For this review, take the finished solid that the model builds, in its own axes (mm). A direction names the side the tool comes from. Coordinates: 2 decimals unless noted, no trailing zeros. Loops run counter-clockwise (first coordinate to the right, second up) from the corner with the lowest first, then second, coordinate; pieces in that order, holes last. Notation, with made-up numbers: (38.5, 1.25) - (88.5, 1.25) arc R24 ccw to (88.5, 20.25) - close; hole circle Ø6 at (6.25, 71.25). An arc over 180 degrees is marked (long way). Use one line per item in the form item = value. Start each with the question number.
1. Draft analysis for pull direction Y (two halves, no side actions). For faces 1 (the face through (28, -33, 0)), 2 (the face through (4, -70, 0)), 3 (the face through (1.267, -65.07, 1.341)), 4 (the face through (11, 6, 0)), state which applies: +Y half, -Y half, draft (parallel to the pull), parting line (faces both ways), or undercut.
2. To check wall thickness, follow probe 1 along X at (y, z) = (-17.5, 0.25); probe 2 along Y at (x, z) = (16, 6); probe 3 along Y at (x, z) = (5, -5.75). State the ranges of each line that lie inside material, in increasing order.
3. Add section A-A on x = 4.5. Give the boundary of the cut face in (y, z), and give its area (3 significant figures).
4. For pin 1 Ø1.5 at (x, z) = (5, 2.5) entering from +Y; pin 2 Ø6 at (y, z) = (-23.5, 4) entering from -X; pin 3 Ø4 at (x, z) = (-3.5, 0.5) entering from -Y, all flat-tipped, find the tip position at first contact; note any pin that passes through.
5. Machinability: for faces 5 (the face through (18, -40, 0)), 6 (the face through (0, -72, 0)), 7 (the face through (23, -24, 0)), which of the approach directions +Z, -Z, +X, -X, +Y, -Y give a long, thin tool a straight path to every point of the face, cutting with its end or side? Answer none if there is none.
6. Add section B-B on z = 0. Count the separate pieces of the cut face and the enclosed holes in it, and give its area (3 significant figures).
7. Add section D-D on y = -64.5. Give the boundary of the cut face in (x, z).
8. Add section C-C on y = -77.5. Give the boundary of the cut face in (x, z).
```python
from build123d import *

# Parameters (mm, degrees)
BOSS_EXTRUDE1_DEPTH          = 7.5
CUT_EXTRUDE1_REACH           = 158.924
SKETCH2_W                    = 18
SKETCH2_H                    = 40
M5_CLEARANCE_HOLE1_D         = 5.8
CUT_EXTRUDE2_REACH           = 158.924
F_7_0_7_DIAMETER_HOLE1_D     = 7
F_7_0_7_DIAMETER_HOLE1_DEPTH = 20
MOVE_FACE1_BY                = 0.6
CUT_EXTRUDE3_REACH           = 141.732
SKETCH14_W                   = 15
SKETCH14_H                   = 15
BOSS_EXTRUDE2_DEPTH          = 10
M5_CLEARANCE_HOLE2_D         = 5.8
SKETCH18_W                   = 33
SKETCH18_H                   = 15
SKETCH18_R                   = 5
BOSS_EXTRUDE3_DEPTH          = 6
SKETCH19_R                   = 5
SKETCH19_R_2                 = 2.9
BOSS_EXTRUDE4_DEPTH          = 1
F_7_0_7_DIAMETER_HOLE2_D     = 7
F_7_0_7_DIAMETER_HOLE2_DEPTH = 30


with BuildPart() as part:
    # Sketch1 → Boss-Extrude1 (new, symmetric)
    with BuildSketch(Plane.XY):
        Polygon((0, 0), (120, 0), (0, -100), align=None)
    extrude(amount=BOSS_EXTRUDE1_DEPTH, both=True)

    # Sketch2 → Cut-Extrude1 (cut, up to next)
    with BuildSketch(Plane.XY.offset(7.5), mode=Mode.PRIVATE) as cut_extrude1_sk1:
        with Locations((9, -40)):
            Rectangle(SKETCH2_W, SKETCH2_H)
    cut_extrude1_tool1 = extrude(cut_extrude1_sk1.sketch, amount=-CUT_EXTRUDE1_REACH, mode=Mode.PRIVATE) & part.part
    add(cut_extrude1_tool1.solids().sort_by_distance((9, -40, 7.5))[0], mode=Mode.SUBTRACT)

    # M5 Clearance Hole1 (through all)
    with Locations(Plane(origin=(0, 0, 0), x_dir=(1, 0, 0), z_dir=(0, 1, 0))):
        with Locations((4.5, 0)):
            Hole(M5_CLEARANCE_HOLE1_D / 2)

    # Sketch8 → Cut-Extrude2 (cut, up to next)
    with BuildSketch(Plane.XY.offset(7.5), mode=Mode.PRIVATE) as cut_extrude2_sk1:
        Polygon((0, -70), (36, -70), (0, -100), align=None)
    cut_extrude2_tool1 = extrude(cut_extrude2_sk1.sketch, amount=-CUT_EXTRUDE2_REACH, mode=Mode.PRIVATE) & part.part
    add(cut_extrude2_tool1.solids().sort_by_distance((12, -80, 7.5))[0], mode=Mode.SUBTRACT)

    # Ø7.0 (7) Diameter Hole1
    with Locations(Plane(origin=(0, 0, 0), x_dir=(1, 0, 0), z_dir=(0, 1, 0))):
        with Locations((60, 0)):
            Hole(F_7_0_7_DIAMETER_HOLE1_D / 2, depth=F_7_0_7_DIAMETER_HOLE1_DEPTH)

    # Move Face1: a curved face moved inward by 0.6
    add(Solid.thicken(part.faces().sort_by_distance((7.4, -65, 0))[0], -MOVE_FACE1_BY), mode=Mode.SUBTRACT)

    # Sketch13 → Cut-Extrude3 (cut, up to next)
    with BuildSketch(Plane.XY.offset(7.5), mode=Mode.PRIVATE) as cut_extrude3_sk1:
        Polygon((28, 0), (28, -70), (36, -70), (120, 0), align=None)
    cut_extrude3_tool1 = extrude(cut_extrude3_sk1.sketch, amount=-CUT_EXTRUDE3_REACH, mode=Mode.PRIVATE) & part.part
    add(cut_extrude3_tool1.solids().sort_by_distance((58.88, -25.2, 7.5))[0], mode=Mode.SUBTRACT)

    # Sketch14 → Boss-Extrude2 (add)
    with BuildSketch(Plane.ZY):
        with Locations((0, -77.5)):
            Rectangle(SKETCH14_W, SKETCH14_H)
    extrude(amount=-BOSS_EXTRUDE2_DEPTH)

    # M5 Clearance Hole2 (through all)
    with Locations(Plane(origin=(10, 0, 0), x_dir=(0, 0, -1), z_dir=(1, 0, 0))):
        with Locations((0, -77.5)):
            Hole(M5_CLEARANCE_HOLE2_D / 2)



with BuildPart() as body_2:
    # Sketch18 → Boss-Extrude3 (new body)
    with BuildSketch(Plane(origin=(0, 0, 0), x_dir=(1, 0, 0), z_dir=(0, 1, 0))):
        with Locations((11.5, 0)):
            Rectangle(SKETCH18_W, SKETCH18_H)
        with Locations(Location((4.5, 0, 0), (0, 0, 270))):
            Circle(SKETCH18_R, mode=Mode.SUBTRACT)
    extrude(amount=BOSS_EXTRUDE3_DEPTH)


with BuildPart() as part_1:
    add(part.part)

    add(body_2.part)  # Boss-Extrude4 merges body 2
    # Sketch19 → Boss-Extrude4 (add)
    with BuildSketch(Plane(origin=(0, 0, 0), x_dir=(1, 0, 0), z_dir=(0, 1, 0))):
        with Locations(Location((4.5, 0, 0), (0, 0, 270))):
            Circle(SKETCH19_R)
        with Locations(Location((4.5, 0, 0), (0, 0, 270))):
            Circle(SKETCH19_R_2, mode=Mode.SUBTRACT)
    extrude(amount=BOSS_EXTRUDE4_DEPTH)

    # Ø7.0 (7) Diameter Hole2
    with Locations(Plane(origin=(0, 6, 0), x_dir=(1, 0, 0), z_dir=(0, 1, 0))):
        with Locations((23, 0)):
            Hole(F_7_0_7_DIAMETER_HOLE2_D / 2, depth=F_7_0_7_DIAMETER_HOLE2_DEPTH)


solid = part_1.part
```
Conclusion:
q1.face_1 = draft
q1.face_2 = undercut
q1.face_3 = undercut
q1.face_4 = +Y half
q2.probe_1 = 0 to 1.61, 7.39 to 19.51, 26.49 to 28
q2.probe_2 = -70 to -60, -20 to 6
q2.probe_3 = -85 to -60, -20 to 6
q3.outline = (-85, -7.5) - (-60, -7.5) - (-60, -3.5) - (-70, -3.5) - (-70, 3.5) - (-60, 3.5) - (-60, 7.5) - (-85, 7.5) - close; (-20, -7.5) - (6, -7.5) - (6, -5) - (1, -5) - (1, -2.9) - (-20, -2.9) - close; (-20, 2.9) - (1, 2.9) - (1, 5) - (6, 5) - (6, 7.5) - (-20, 7.5) - close; hole circle Ø5.8 at (-77.5, 0)
q3.area = 497 mm^2
q4.pin_1 = 1
q4.pin_2 = 18
q4.pin_3 = 0
q5.face_5 = +Z, -Z, -X
q5.face_6 = +Z, -Z, -X, -Y
q5.face_7 = +Y
q6.separate_pieces = 3
q6.enclosed_holes = 0
q6.area = 1,080 mm^2
q7.outline = (0, -7.5) - (28, -7.5) - (28, 7.5) - (0, 7.5) - close; hole circle Ø7 at (4.5, 0)
q8.outline = (0, -7.5) - (10, -7.5) - (10, -2.9) - (0, -2.9) - close; (0, 2.9) - (10, 2.9) - (10, 7.5) - (0, 7.5) - close
